Verification items for the finished model (mm, model axes). Face numbers are marked on the shaded views. A direction names the side the tool comes from. Give positions to 0.01 mm unless a question says otherwise; leave off trailing zeros.
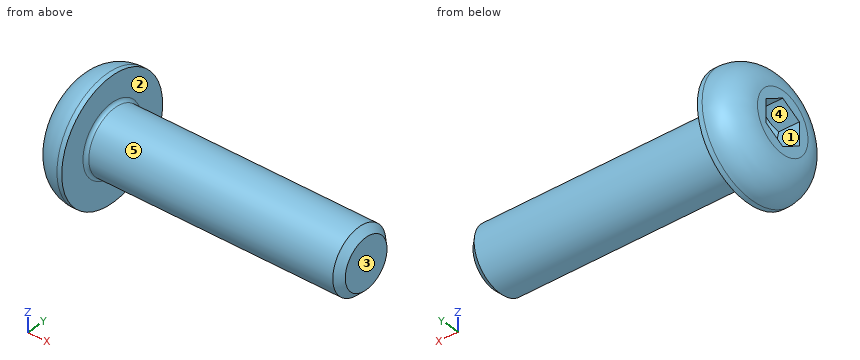
Autodesk Inventor part; units mm, degrees
ref_plane "Work Plane1" through (30, 0, 0) normal (0, -0.5, 0.866) x (1, 0, 0)
ref_plane "YZ Plane" through (0, 0, 0) normal (1, 0, 0) x (0, 1, 0)
ref_plane "XZ Plane" through (0, 0, 0) normal (0, 1, 0) x (-1, 0, 0)
sketch "Esquisse1" plane through (0, 0, 0) normal (0, 0, 1) x (1, 0, 0)
  line L0 (-0.0667, 0) -> (16, 0)
  line L1 (16, 0) -> (16, 2)
  line L2 (16, 2) -> (1.4, 2)
  line L3 (1.4, 2) -> (0.9706, 2)
  line L4 (0.9706, 2) -> (0, 2)
  line L5 (0, 2) -> (0, 3.8)
  line L6 (0, 3.8) -> (-2.2, 3.8)
  line L7 (-2.2, 3.8) -> (-2.2, 1.4434)
  line L8 (-2.2, 1.4434) -> (-0.9, 1.4434)
  line L9 (-0.9, 1.4434) -> (-0.0667, 0)
  line L10 (-5.84, 0) -> (19.64, 0)
  line L11 (0, -0.76) -> (0, 4.56)
  line L12 (1.4, 2) -> (0, 2) construction
  dimension "d0" = 14.6
  dimension "d1" = 0.4294
  dimension "d2" = 2.2
  dimension "d3" = 1.3
  dimension "d4" = 60
  dimension "d5" = 4
  dimension "d6" = 4
  dimension "d7" = 2.8868
  dimension "d8" = 7.6
  dimension "d19" = 16
revolve "Corps" add sketch "Esquisse1" angle 360 about axis through (-0.0667, 0, 0) along (1, 0, 0)
sketch "Esquisse2" plane through (-2.2, 0, 0) normal (-1, 0, 0) x (0, 0, 1)
  circle A0 centre (0, 0) radius 1.4434
  line L0 (0, -5.32) -> (0, 5.32)
  line L1 (-5.32, 0) -> (5.32, 0)
  line L2 (1.4434, 0) -> (0.7217, -1.25)
  line L3 (0.7217, -1.25) -> (-0.7217, -1.25)
  line L4 (-0.7217, -1.25) -> (-1.4434, 0)
  line L5 (-1.4434, 0) -> (-0.7217, 1.25)
  line L6 (-0.7217, 1.25) -> (0.7217, 1.25)
  line L7 (0.7217, 1.25) -> (1.4434, 0)
  point P0 (0, 0)
extrude "Rainure" add sketch "Esquisse2" against normal up to next contours L7 A0 | A0 L2 | L6 L0 A0 | A0 L0 L3 | L0 L6 A0 | A0 L3 L0 | L4 A0 | A0 L5
fillet "Congé1" radius 1.9 1 edges at (-2.2, -3.8, 0)
thread "Filetage"
chamfer "Chanfrein1" distance 0.4294 distance2 0.4294 1 edges at (16, -2, 0) measured on face at (16, 0.527, -0.2661)
fillet "Congé2" radius 0.2 1 edges at (0, -2, 0)
ref_plane "Work Plane1" through (30, 0, 0) normal (0, -0.5, 0.866) x (1, 0, 0)
equation "\"d0\" = GEL"
equation "\"d1\" = GAL"
equation "\"d2\" = KOH"
equation "\"d3\" = INTI"
equation "\"d5\" = GD"
equation "\"d6\" = BDM"
equation "\"d7\" = 1.1547 * SW"
equation "\"d8\" = KOD"
equation "\"d19\" = NLG"
equation "\"d16\" = RR"
equation "\"d12\" = GEL"
equation "\"d14\" = -0.5 * SPD + 0.5 * GD"
equation "\"d15\" = GUL"
equation "\"d29\" = R"
equation "\"GD\" = NND"
equation "\"NLG\" = 16"
equation "\"GEL\" = 14.6"
equation "\"KOD\" = 7.6"
equation "\"KOH\" = 2.2"
equation "\"INTI\" = 1.3"
equation "\"GAL\" = 0.61345 * PTC"
equation "\"GUL\" = 0.61345 * PTC"
equation "\"BDM\" = NND"
equation "\"SW\" = 2.5"
equation "\"RR\" = 1.9"
equation "\"SPD\" = 3.14117"
equation "\"d28\" = R"
equation "\"R\" = 0.2"
equation "\"TOA\" = 30deg"
equation "\"THREADDIA\" = 4"
equation "\"KOD1\" = KOD - 2 * RR"
equation "\"PTC\" = 0.7"
equation "\"NND\" = 4"
equation "\"E0\" = 1.155 * SW"
equation "\"GD1\" = THREADDIA - 1.2269 * PTC"
properties part number "ANSI B18.3.4M - M4 x 0.7 x 16" material "Acier, doux"
(1) Release check for a two-part mould opening along Z. For the marked faces 3, 4 and 5 record: pulls with the +Z half, pulls with the -Z half, needs draft (parallel to the pull), parting line crosses it, or undercut.
Solved:
face 3: needs draft
face 4: undercut
face 5: parting line crosses it
(2) Set-up check for the marked faces 1 and 2: record each of +Z, -Z, +X, -X, +Y, -Y from which the full face is reachable in a straight line by a thin tool's end or side.
Solved:
face 1: -X
face 2: +X
(3) Go/stop test with flat-tipped pins: pin 1 (3 mm diameter, centred on x = 0.5, y = 2.5, fed in from +Z); pin 2 (1.6 mm diameter, centred on x = -1.5, z = 0, fed in from -Y). Record where each tip stops, or that it passes through.
Solved:
pin 1: stops at z = 3.64
pin 2: stops at y = -3.76
(4) Scan lines: line 1 (Z direction, x = 5.5, y = 0); line 2 (X direction, y = 1, z = 2); line 3 (X direction, y = -3, z = 1.5). Record each from-to range of solid material in increasing order.
Solved:
line 1: z = -2 to 2
line 2: x = -2.17 to 0
line 3: x = -1.52 to 0
